For this review, take the finished solid that the model builds, in its own axes (mm). A direction names the side the tool comes from. Give positions to 0.01 mm unless a question says otherwise; leave off trailing zeros. Order: outer loops, then holes, each group sorted by start corner. A loop starts at its lowest first (then second) coordinate and runs counter-clockwise, first axis right, second up. Notation, with made-up numbers: (58, 27) -> (69, 27) arc R22 ccw to (69, 56) -> close; hole circle Ø5 at (21.5, -1). An arc over 180 degrees is marked (long way). Return JSON: item names as keys, results as strings. Group by question number.
1) Insertion check: P1, Ø9.5, axis at x = 1305, z = -25, coming from the +Y side; P2, Ø5, axis at x = 1055, z = -25, coming from the -Y side. Each pin has a flat end and moves straight along its axis. Give the tip position at first contact, or say it passes through.
2) To check wall thickness, follow line 1 along Y through (x, z) = (932, -4.5); line 2 along Z through (x, y) = (981, -15); line 3 along Z through (x, y) = (1105, -18). State the ranges of each line that lie inside material, in increasing order.
3) For faces 5 (the face through (0, -18, -3)), 6 (the face through (740, 0, -37)), list the 3-axis set-ups (+Z, -Z, +X, -X, +Y, -Y) from which the entire face can be reached by the end or side of a thin tool; tool diameter is ignored.
4) The part is to be moulded in two halves that separate along Z. For faces 1 (the face through (740, 20, 1)), 2 (the face through (740, -17, 1)), 3 (the face through (740, 17, 1)), 4 (the face through (740, 0, -40)), say which applies: released by +Z, released by -Z, zero draft, split by the parting line, or undercut.
5) Add section A-A (x = 430.5). Give the boundary of the cut face in (y, z).
6) Add section B-B (z = 1). Give the boundary of the cut face in (x, y), then the cut area to 3 significant figures.
7) Add section C-C (y = -7). Give the boundary of the cut face in (x, z), then the cut area to 3 significant figures.
from build123d import *

# Parameters (mm, degrees)
SKETCH_1_W          = 74
SKETCH_1_H          = 34
EXTRUDE_1_DEPTH     = 1500
SKETCH_2_R          = 4.05
CUT_EXTRUDE_1_DEPTH = 41


with BuildPart() as part:
    # Эскиз1 → Вытянуть-Тонкостенный1 (new body)
    with BuildSketch(Plane(origin=(0, 0, 0), x_dir=(0, 0, -1), z_dir=(1, 0, 0))):
        with BuildLine():
            Line((40, 17), (40, -17))
            ThreePointArc((40, -17), (39.121320344, -19.121320344), (37, -20))
            Line((37, -20), (-37, -20))
            ThreePointArc((-37, -20), (-39.121320344, -19.121320344), (-40, -17))
            Line((-40, -17), (-40, 17))
            ThreePointArc((-40, 17), (-39.121320344, 19.121320344), (-37, 20))
            Line((-37, 20), (37, 20))
            ThreePointArc((37, 20), (39.121320344, 19.121320344), (40, 17))
        make_face()
        Rectangle(SKETCH_1_W, SKETCH_1_H, mode=Mode.SUBTRACT)
    extrude(amount=EXTRUDE_1_DEPTH)

    # Эскиз2 → Вырез-Вытянуть1 (cut, through all)
    with BuildSketch(Plane(origin=(0, 20, 0), x_dir=(1, 0, 0), z_dir=(0, 1, 0))):
        with Locations((1455, -25)):
            Circle(SKETCH_2_R)
        with Locations((1405, -25)):
            Circle(SKETCH_2_R)
        with Locations((1355, -25)):
            Circle(SKETCH_2_R)
        with Locations((1305, -25)):
            Circle(SKETCH_2_R)
        with Locations((1155, -25)):
            Circle(SKETCH_2_R)
        with Locations((1105, -25)):
            Circle(SKETCH_2_R)
        with Locations((1055, -25)):
            Circle(SKETCH_2_R)
        with Locations((1005, -25)):
            Circle(SKETCH_2_R)
        with Locations((1005, 25)):
            Circle(SKETCH_2_R)
        with Locations((1055, 25)):
            Circle(SKETCH_2_R)
        with Locations((1105, 25)):
            Circle(SKETCH_2_R)
        with Locations((1155, 25)):
            Circle(SKETCH_2_R)
        with Locations((1305, 25)):
            Circle(SKETCH_2_R)
        with Locations((1355, 25)):
            Circle(SKETCH_2_R)
        with Locations((1405, 25)):
            Circle(SKETCH_2_R)
        with Locations((1455, 25)):
            Circle(SKETCH_2_R)
    extrude(amount=-CUT_EXTRUDE_1_DEPTH, mode=Mode.SUBTRACT)


solid = part.part
Evaluation:
{
 "1": {"P1": "y = 20", "P2": "through"},
 "2": {"line 1": "-20 to -17, 17 to 20", "line 2": "-40 to -37, 37 to 40", "line 3": "-39.83 to -29.05, -20.95 to 20.95, 29.05 to 39.83"},
 "3": {"face 5": "+Z, -Z, -X, +Y, -Y", "face 6": "+X, -X"},
 "4": {"face 1": "zero draft", "face 2": "undercut", "face 3": "undercut", "face 4": "released by -Z"},
 "5": {"outline": "(-20, -37) arc R3 ccw to (-17, -40) -> (17, -40) arc R3 ccw to (20, -37) -> (20, 37) arc R3 ccw to (17, 40) -> (-17, 40) arc R3 ccw to (-20, 37) -> close; hole (-17, -37) -> (17, -37) -> (17, 37) -> (-17, 37) -> close"},
 "6": {"outline": "(0, -20) -> (1500, -20) -> (1500, -17) -> (0, -17) -> close; (0, 17) -> (1500, 17) -> (1500, 20) -> (0, 20) -> close", "area": "9,000 mm^2"},
 "7": {"outline": "(0, -40) -> (1500, -40) -> (1500, -37) -> (0, -37) -> close; (0, 37) -> (1500, 37) -> (1500, 40) -> (0, 40) -> close", "area": "9,000 mm^2"}
}
